Autodesk Fusion 360 part; units mm, degrees
sketch "Sketch1" plane through (0, 0, 0) normal (0, 1, 0) x (1, 0, 0)
  line L0 (0, 0) -> (30, 0)
  line L1 (30, 0) -> (30, -12.8)
  line L2 (30, -12.8) -> (0, -12.8)
  line L3 (0, -12.8) -> (0, 0)
  dimension "d1" = 30
  dimension "d2" = 12.8
extrude "Extrude1" add sketch "Sketch1" along normal blind 12.8
sketch "Sketch2" plane through (0, 12.8, 0) normal (0, 1, 0) x (-1, 0, 0)
  line L0 (0, 12.8) -> (-30, 12.8)
  line L1 (-30, 12.8) -> (-30, 0)
  line L2 (-30, 0) -> (0, 0)
  line L3 (0, 0) -> (0, 12.8)
  line L4 (-15, 0) -> (-15, 12.8) construction
  line L5 (0, 6.4) -> (-30, 6.4) construction
  point P0 (-15, 6.4)
hole "Hole1" at (15, 12.8, 6.4) direction (0, -1, 0) diameter 2.5 end through all
sketch "Sketch3" plane through (0, 0, 12.8) normal (0, 0, 1) x (1, 0, 0)
  line L0 (0, 0) -> (30, 0)
  line L1 (30, 0) -> (30, 12.8)
  line L2 (30, 12.8) -> (0, 12.8)
  line L3 (0, 12.8) -> (0, 0)
  line L4 (0, 6.4) -> (30, 6.4) construction
  point P0 (5, 6.4)
  point P1 (15, 6.4)
  dimension "d8" = 10
  dimension "d9" = 5
hole "Hole2" at (10, 6.4, 12.8) direction (0, 0, -1) diameter 2.5 end through all
hole "Hole3" at (20, 6.4, 12.8) direction (0, 0, -1) diameter 2.5 end through all
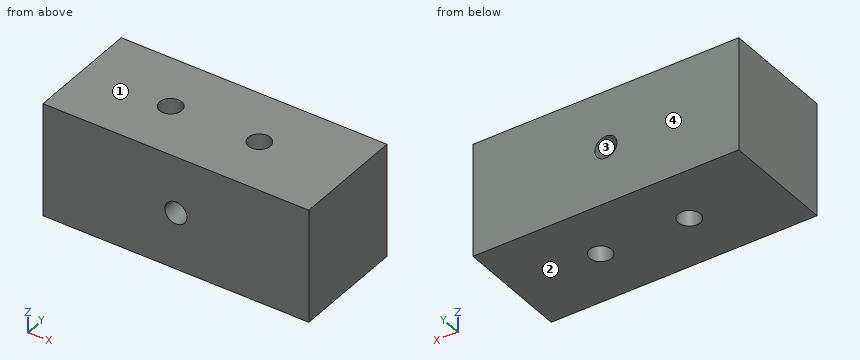
The model under review builds one solid part; all positions refer to its coordinate system, in mm. Face numbers are marked on the shaded views. Give positions to 0.01 mm unless a question says otherwise; leave off trailing zeros. Order: outer loops, then holes, each group sorted by start corner. A loop starts at its lowest first (then second) coordinate and runs counter-clockwise, first axis right, second up. Notation, with made-up numbers: M 68,-15.5 L 99,-15.5 A13 cw 99,4.5 Z; hole C -5,-40 d8. An arc over 180 degrees is marked long. Answer in a Markdown table with one row per item. Add a question column.
1. Add section D-D on z = 2.5. State the section outline as (x, y) points, plus the area to 3 significant figures.
2. Add section C-C on x = 15. State the section outline as (y, z) points.
3. For pin 1 Ø2 at (x, y) = (10, 6.4) entering from -Z, flat-tipped, find the tip position at first contact; note if it passes through.
4. Mouldability with a two-part tool opening along Z and no side actions: class the marked faces 1, 2, 3 and 4 as released by +Z, released by -Z, zero draft, split by the parting line, or undercut.
5. Add section B-B on y = 6.4. State the section outline as (x, z) points.
6. To check wall thickness, follow line 1 along Z through (x, y) = (15, 5.5); line 2 along X through (y, z) = (6.4, 3.25). State the ranges of each line that lie inside material, in increasing order.
7. Add section A-A on z = 6.4. State the section outline as (x, y) points.
The answers:
| question | item | result |
|---|---|---|
| 1 | outline | M 0,0 L 30,0 L 30,12.8 L 0,12.8 Z; hole C 10,6.4 d2.5; hole C 20,6.4 d2.5 |
| 1 | area | 374 mm2 |
| 2 | outline | M 0,0 L 12.8,0 L 12.8,5.15 L 0,5.15 Z; M 0,7.65 L 12.8,7.65 L 12.8,12.8 L 0,12.8 Z |
| 3 | pin 1 | through |
| 4 | face 1 | released by +Z |
| 4 | face 2 | released by -Z |
| 4 | face 3 | undercut |
| 4 | face 4 | zero draft |
| 5 | outline | M 0,0 L 8.75,0 L 8.75,12.8 L 0,12.8 Z; M 11.25,0 L 18.75,0 L 18.75,12.8 L 11.25,12.8 Z; M 21.25,0 L 30,0 L 30,12.8 L 21.25,12.8 Z; hole C 15,6.4 d2.5 |
| 6 | line 1 | 0 to 5.15, 7.65 to 12.8 |
| 6 | line 2 | 0 to 8.75, 11.25 to 18.75, 21.25 to 30 |
| 7 | outline | M 0,0 L 13.75,0 L 13.75,12.8 L 0,12.8 Z; M 16.25,0 L 30,0 L 30,12.8 L 16.25,12.8 Z; hole C 10,6.4 d2.5; hole C 20,6.4 d2.5 |
